```python
from build123d import *

# Parameters (mm, degrees)
F0_R     = 1.8
F0_R_2   = 11.1
F0_R_3   = 3.2
F2_DEPTH = 4.3
F3_DEPTH = 1.7
F4_DEPTH = 16.8
F5_R     = 3
F5_R_2   = 2
F6_DEPTH = 42.401
F5_R_3   = 3.75
F7_DEPTH = 2.8


with BuildPart() as f2:
    # F0 (on Front) → F2 (new body, through all)
    with BuildSketch(Plane.XZ):
        with BuildLine():
            ThreePointArc((-19.2, -11.8), (-20.614214, -12.385786), (-21.2, -13.8))
            Line((-21.2, -13.8), (-21.2, -19.2))
            ThreePointArc((-21.2, -19.2), (-20.614214, -20.614214), (-19.2, -21.2))
            Line((-19.2, -21.2), (19.2, -21.2))
            ThreePointArc((19.2, -21.2), (20.614214, -20.614214), (21.2, -19.2))
            Line((21.2, -19.2), (21.2, -13.8))
            ThreePointArc((21.2, -13.8), (20.614214, -12.385786), (19.2, -11.8))
            Line((19.2, -11.8), (-19.2, -11.8))
        make_face()
        with Locations((-14.9, -14.9)):
            Circle(F0_R, mode=Mode.SUBTRACT)
        with Locations((14.9, -14.9)):
            Circle(F0_R, mode=Mode.SUBTRACT)
        with BuildLine():
            Line((19.2, 21.2), (-19.2, 21.2))
            ThreePointArc((-19.2, 21.2), (-20.614214, 20.614214), (-21.2, 19.2))
            Line((-21.2, 19.2), (-21.2, -13.8))
            ThreePointArc((-21.2, -13.8), (-20.614214, -12.385786), (-19.2, -11.8))
            Line((-19.2, -11.8), (19.2, -11.8))
            ThreePointArc((19.2, -11.8), (20.614214, -12.385786), (21.2, -13.8))
            Line((21.2, -13.8), (21.2, 19.2))
            ThreePointArc((21.2, 19.2), (20.614214, 20.614214), (19.2, 21.2))
        make_face()
        with Locations((-14.9, 14.9)):
            Circle(F0_R, mode=Mode.SUBTRACT)
        Circle(F0_R_2, mode=Mode.SUBTRACT)
        with Locations((14.9, 14.9)):
            Circle(F0_R_3, mode=Mode.SUBTRACT)
    extrude(amount=F2_DEPTH)

    # F0 (on Front) → F3 (join, through all)
    with BuildSketch(Plane.XZ):
        with Locations((14.9, 14.9)):
            Circle(F0_R_3)
        with Locations((14.9, 14.9)):
            Circle(F0_R, mode=Mode.SUBTRACT)
    extrude(amount=F3_DEPTH)

    # F0 (on Front) → F4 (join, through all)
    with BuildSketch(Plane.XZ):
        with BuildLine():
            ThreePointArc((-19.2, -11.8), (-20.614214, -12.385786), (-21.2, -13.8))
            Line((-21.2, -13.8), (-21.2, -19.2))
            ThreePointArc((-21.2, -19.2), (-20.614214, -20.614214), (-19.2, -21.2))
            Line((-19.2, -21.2), (19.2, -21.2))
            ThreePointArc((19.2, -21.2), (20.614214, -20.614214), (21.2, -19.2))
            Line((21.2, -19.2), (21.2, -13.8))
            ThreePointArc((21.2, -13.8), (20.614214, -12.385786), (19.2, -11.8))
            Line((19.2, -11.8), (-19.2, -11.8))
        make_face()
        with Locations((-14.9, -14.9)):
            Circle(F0_R, mode=Mode.SUBTRACT)
        with Locations((14.9, -14.9)):
            Circle(F0_R, mode=Mode.SUBTRACT)
    extrude(amount=F4_DEPTH)

    # F5 (on face) → F6 (cut, through all)
    with BuildSketch(Plane(origin=(0, 0, -21.2), x_dir=(1, 0, 0), z_dir=(0, 0, -1))):
        with Locations((-6.2, 10.55)):
            Circle(F5_R)
        with Locations((11.2, 10.55)):
            Circle(F5_R_2)
    extrude(amount=-F6_DEPTH, mode=Mode.SUBTRACT)

    # F5 (on face) → F7 (cut, through all)
    with BuildSketch(Plane(origin=(0, 0, -21.2), x_dir=(1, 0, 0), z_dir=(0, 0, -1))):
        with Locations((11.2, 10.55)):
            Circle(F5_R_3)
        with Locations((11.2, 10.55)):
            Circle(F5_R_2, mode=Mode.SUBTRACT)
    extrude(amount=-F7_DEPTH, mode=Mode.SUBTRACT)


solid = f2.part
```
Can you work these out from the model? Positions are in its coordinate system, mm. A direction names the side the tool comes from. Round coordinates to 2 decimals unless told otherwise and drop trailing zeros. Loops run counter-clockwise (first coordinate to the right, second up) from the corner with the lowest first, then second, coordinate; pieces in that order, holes last. Notation, with made-up numbers: (43, 54.25) -> (70, 54.25) arc R26 cw to (70, 82.25) -> close; hole circle Ø11 at (80, 42). An arc over 180 degrees is marked (long way). Answer in a Markdown table with one row per item.
Item 1: Suppose I cut it at A-A, the plane x = 0. List the corners of the cut face in (y, z) for me.
Answer block:
| item | result |
|---|---|
| outline | (-16.8, -21.2) -> (0, -21.2) -> (0, -11.1) -> (-4.3, -11.1) -> (-4.3, -11.8) -> (-16.8, -11.8) -> close; (-4.3, 11.1) -> (0, 11.1) -> (0, 21.2) -> (-4.3, 21.2) -> close |
Item 2: Suppose I cut it at C-C, the plane y = -2.25. List the corners of the cut face in (x, z) for me.
Answer block:
| item | result |
|---|---|
| outline | (-21.2, -19.2) arc R2 ccw to (-19.2, -21.2) -> (19.2, -21.2) arc R2 ccw to (21.2, -19.2) -> (21.2, 19.2) arc R2 ccw to (19.2, 21.2) -> (-19.2, 21.2) arc R2 ccw to (-21.2, 19.2) -> close; hole circle Ø3.6 at (-14.9, -14.9); hole circle Ø3.6 at (-14.9, 14.9); hole circle Ø22.2 at (0, 0); hole circle Ø6.4 at (14.9, 14.9); hole circle Ø3.6 at (14.9, -14.9) |
Item 3: Suppose I cut it at B-B, the plane z = -14.9. List the corners of the cut face in (x, y) for me.
Answer block:
| item | result |
|---|---|
| outline | (-21.2, -16.8) -> (-16.7, -16.8) -> (-16.7, 0) -> (-21.2, 0) -> close; (-13.1, -16.8) -> (13.1, -16.8) -> (13.1, -11.17) arc R2 cw (long way) to (13.1, -9.93) -> (13.1, 0) -> (-13.1, 0) -> close; (16.7, -16.8) -> (21.2, -16.8) -> (21.2, 0) -> (16.7, 0) -> close; hole circle Ø6 at (-6.2, -10.55) |
Item 4: Suppose I cut it at D-D, the plane z = 0. List the corners of the cut face in (x, y) for me.
Answer block:
| item | result |
|---|---|
| outline | (-21.2, -4.3) -> (-11.1, -4.3) -> (-11.1, 0) -> (-21.2, 0) -> close; (11.1, -4.3) -> (21.2, -4.3) -> (21.2, 0) -> (11.1, 0) -> close |
Item 5: Will these pins go through, and if not, where does the flat tip stop? P1, Ø1.9, axis at x = 16, z = 14, coming from the -Y side; P2, Ø10.5, axis at x = 10.5, z = -4.5, coming from the -Y side; P3, Ø8.5, axis at x = 11.2, y = -10.55, coming from the +Z side.
Answer block:
| item | result |
|---|---|
| P1 | y = -1.7 |
| P2 | y = -4.3 |
| P3 | z = -11.8 |
Item 6: If I drill on probe 1 along Z at (x, y) = (14.9, -3.4); probe 2 along X at (y, z) = (-1.75, -15), over which ranges is the centre line in solid material (lowest first)?
Answer block:
| item | result |
|---|---|
| probe 1 | -21.2 to -16.7, -13.1 to 11.7, 18.1 to 21.2 |
| probe 2 | -21.2 to -16.7, -13.1 to 13.1, 16.7 to 21.2 |
Item 7: We'd pull the mould along Z, two halves only. Please class faces 4 (the cylindrical face through (20.6, -8.28, -20.63)), 5 (the cylindrical face through (-13.932, -2.12, 16.418)), 6 (the cylindrical face through (-20.6, -10.46, -12.37)), 7 (the cylindrical face through (17.856, -2.982, 13.674)): released by +Z, released by -Z, zero draft, split by the parting line, or undercut.
Answer block:
| item | result |
|---|---|
| face 4 | released by -Z |
| face 5 | undercut |
| face 6 | released by +Z |
| face 7 | undercut |
Item 8: On a 3-axis mill with a long thin cutter (end or side, diameter ignored), from which of +Z, -Z, +X, -X, +Y, -Y can I reach the whole of each face in a straight line? I mean faces 1 (the flat face through (-10, 0, -9)), 2 (the cylindrical face through (20.63, -10.46, -12.4)), 3 (the cylindrical face through (12.93, -7.223, -19.82)). Say none if no direction works.
Answer block:
| item | result |
|---|---|
| face 1 | +Z, -Z, +X, -X, +Y |
| face 2 | +Z, +X, -Y |
| face 3 | -Z |
